Autodesk Inventor part; units mm, degrees
ref_plane "起始平面" through (0, 0, 0) normal (0, 1, 0) x (-1, 0, 0)
ref_plane "终止平面" through (0, 100, 0) normal (0, 1, 0) x (-1, 0, 0)
ref_plane "YZ Plane" through (0, 0, 0) normal (1, 0, 0) x (0, 1, 0)
ref_plane "起始平面" through (0, 0, 0) normal (0, 1, 0) x (-1, 0, 0)
ref_plane "终止平面" through (0, 100, 0) normal (0, 1, 0) x (-1, 0, 0)
sketch "草图" plane through (0, 0, 0) normal (0, 1, 0) x (-1, 0, 0)
  line L0 (-9.1, 10.0192) -> (-9.101, 10.0203)
  line L1 (-10, 10) -> (-9.5607, 9.5607) construction
  arc A0 (-8.5, 10) -> (-10, 8.5) centre (-8.5, 8.5) ccw
  circle A1 centre (0, 0) radius 2.5
  line L2 (-2.9808, 3.9) -> (0, 3.9)
  line L3 (-3.9, 0) -> (-3.9, 2.9808)
  line L4 (-2.5, 0) -> (-3.1, 0)
  line L5 (2.9808, 3.9) -> (0, 3.9)
  circle A2 centre (0, 0) radius 2.5
  circle A3 centre (0, 0) radius 2.5
  circle A4 centre (0, 0) radius 2.5
  line L6 (0, 16.3557) -> (0, -12.0006)
  line L7 (-4.3, 9.1) -> (-4.3, 10)
  line L8 (2.9808, -3.9) -> (0, -3.9)
  line L9 (-3.9, 0) -> (-3.9, -2.9808)
  line L10 (3.9, 0) -> (3.9, -2.9808)
  line L11 (-2.9808, -3.9) -> (-5.5, -6.4192)
  line L12 (-2.9808, -3.9) -> (0, -3.9)
  line L13 (3.8, -8.2) -> (3.8, -9.1)
  line L14 (5.5, -6.4192) -> (2.9808, -3.9)
  line L15 (3.8, -9.1) -> (4.3, -9.1)
  line L16 (5.5, -8.2) -> (3.8, -8.2)
  line L17 (5.5, -8.2) -> (5.5, -6.4192)
  line L18 (3.9, -2.9808) -> (6.4192, -5.5)
  line L19 (8.2, -3.8) -> (8.2, -5.5)
  line L20 (8.2, -5.5) -> (6.4192, -5.5)
  line L21 (8.2, -3.8) -> (9.1, -3.8)
  line L22 (9.1, -3.8) -> (9.1, -4.3)
  line L23 (9.1, -4.3) -> (10, -4.3)
  line L24 (10, -4.3) -> (10, -8.5)
  arc A5 (8.5, -10) -> (10, -8.5) centre (8.5, -8.5) ccw
  line L25 (8.5, -10) -> (4.3, -10)
  line L26 (4.3, -9.1) -> (4.3, -10)
  line L27 (5.5, 6.4192) -> (2.9808, 3.9)
  line L28 (3.9, 2.9808) -> (6.4192, 5.5)
  line L29 (10, 4.3) -> (10, 8.5)
  line L30 (3.9, 0) -> (3.9, 2.9808)
  line L31 (5.5, 8.2) -> (5.5, 6.4192)
  line L32 (5.5, 8.2) -> (3.8, 8.2)
  line L33 (4.3, 9.1) -> (4.3, 10)
  arc A6 (10, 8.5) -> (8.5, 10) centre (8.5, 8.5) ccw
  line L34 (8.5, 10) -> (4.3, 10)
  line L35 (8.2, 3.8) -> (9.1, 3.8)
  line L36 (9.1, 4.3) -> (10, 4.3)
  line L37 (9.1, 3.8) -> (9.1, 4.3)
  line L38 (8.2, 3.8) -> (8.2, 5.5)
  line L39 (8.2, 5.5) -> (6.4192, 5.5)
  line L40 (3.8, 8.2) -> (3.8, 9.1)
  line L41 (3.8, 9.1) -> (4.3, 9.1)
  line L42 (-10, 4.3) -> (-10, 8.5)
  line L43 (-8.5, 10) -> (-4.3, 10)
  line L44 (-9.1, 4.3) -> (-10, 4.3)
  line L45 (-9.1, 3.8) -> (-9.1, 4.3)
  line L46 (-8.2, 3.8) -> (-9.1, 3.8)
  line L47 (-8.2, 5.5) -> (-6.4192, 5.5)
  line L48 (-8.2, 3.8) -> (-8.2, 5.5)
  line L49 (-5.5, 8.2) -> (-5.5, 6.4192)
  line L50 (-3.8, 9.1) -> (-4.3, 9.1)
  line L51 (-3.8, 8.2) -> (-3.8, 9.1)
  line L52 (-5.5, 8.2) -> (-3.8, 8.2)
  line L53 (-3.9, 2.9808) -> (-6.4192, 5.5)
  line L54 (-2.9808, 3.9) -> (-5.5, 6.4192)
  line L55 (-5.5, -8.2) -> (-3.8, -8.2)
  line L56 (-5.5, -8.2) -> (-5.5, -6.4192)
  line L57 (-3.9, -2.9808) -> (-6.4192, -5.5)
  line L58 (-3.8, -8.2) -> (-3.8, -9.1)
  line L59 (-3.8, -9.1) -> (-4.3, -9.1)
  line L60 (-4.3, -9.1) -> (-4.3, -10)
  line L61 (-8.2, -5.5) -> (-6.4192, -5.5)
  line L62 (-8.2, -3.8) -> (-9.1, -3.8)
  line L63 (-9.1, -3.8) -> (-9.1, -4.3)
  line L64 (-8.5, -10) -> (-4.3, -10)
  line L65 (-9.1, -4.3) -> (-10, -4.3)
  line L66 (-10, -4.3) -> (-10, -8.5)
  arc A7 (-10, -8.5) -> (-8.5, -10) centre (-8.5, -8.5) ccw
  line L67 (-8.2, -3.8) -> (-8.2, -5.5)
  dimension "圆角" = 1.5
  dimension "宽度" = 20
extrude "实体" add sketch "草图" along normal up to surface (100 mm away) from surface at 0 contours L43 L7 L50 L51 L52 L49 L54 L2 L6 A1 L12 L11 L56 L55 L58 L59 L60 L64 A7 L66 L65 L63 L62 L67 L61 L57 L9 L3 L53 L47 L48 L46 L45 L44 L42 A0 | L5 L27 L31 L32 L40 L41 L33 L34 A6 L29 L36 L37 L35 L38 L39 L28 L30 L10 L18 L20 L19 L21 L22 L23 L24 A5 L25 L26 L15 L13 L16 L17 L14 L8 L6 A1
sketch "草图2" plane through (0, 0, 0) normal (0, 1, 0) x (-1, 0, 0)
  line L0 (0, 0) -> (10, 0)
ref_plane "工作平面3" through (0, 0, 0) normal (0, 0, -1) x (-1, 0, 0)
sketch "草图3" plane through (0, 0, 0) normal (0, 0, -1) x (-1, 0, 0)
  line L0 (-2, 0) -> (12, 0)
  line L1 (-2, 100) -> (12, 100)
  dimension "d11" = 100
equation "\"G_OFFSET_START\" = 0"
equation "\"G_OFFSET_END\" = 0"
equation "\"G_L\" = d11"
properties part number "欧标 2020铝合金钢材-01"
Can you work these out from the model? Positions are in its coordinate system, mm. A direction names the side the tool comes from. Give positions to 0.01 mm unless a question says otherwise; leave off trailing zeros. Write each loop counter-clockwise with the first axis right and the second up, starting at its lowest first coordinate (ties: lowest second). Pieces come first, ordered by that corner, then holes. Notation, with made-up numbers: (37, 58.25) -> (90, 58.25) arc R25 ccw to (90, 76.25) -> close; hole circle Ø3 at (56.5, 84). An arc over 180 degrees is marked (long way). Answer as a JSON object with one key per item and string values. Group by question number.
Item 1: For faces 1 (the face through (5.5, 49, -7)), 2 (the face through (10, 49, -6)), 3 (the face through (0, 49, -3.9)), 4 (the face through (-3.9, 49, 0)), which set-ups out of +Z, -Z, +X, -X, +Y, -Y let a thin tool reach every point of the face, with its end or its side?
Item 2: Suppose I cut it at B-B (x = 0). Please give me the cut outline in (y, z).
Item 3: Please list where these lines run through material, in increasing order: line 1 (X direction, y = 39.5, z = 0); line 2 (Z direction, x = 8.5, y = 89); line 3 (Z direction, x = 5.25, y = 60). Write a range as [from, to].
Item 4: I'm going to push flat-ended pins straight in: P1, Ø1.5, axis at y = 52.5, z = 1.5, coming from the -X side; P2, Ø2, axis at x = -3, z = 3.5, coming from the -Y side; P3, Ø5, axis at x = -1, y = 34.5, coming from the -Z side; P4, Ø0.5, axis at y = 27, z = -9.5, coming from the +X side. Where does each tip first touch, or does it pass through?
Item 5: We'd pull the mould along Z, two halves only. Please class faces 5 (the face through (-4.26, 49.3, 5.18)), 6 (the face through (-10, 49, -6)), 7 (the face through (0, 49, 3.9)): +Z half, -Z half, draft (parallel to the pull), parting line (faces both ways), or undercut.
Item 6: Suppose I cut it at A-A (z = 1.5). Please give me the cut outline in (x, y), plus the area to 3 significant figures.
Findings:
{
 "1": {"face 1": "+Y, -Y", "face 2": "+Z, -Z, +X, +Y, -Y", "face 3": "-Z, +Y, -Y", "face 4": "-X, +Y, -Y"},
 "2": {"outline": "(0, -3.9) -> (100, -3.9) -> (100, -2.5) -> (0, -2.5) -> close; (0, 2.5) -> (100, 2.5) -> (100, 3.9) -> (0, 3.9) -> close"},
 "3": {"line 1": "x = [-3.9, -2.5], [2.5, 3.9]", "line 2": "z = [-10, -3.8], [3.8, 10]", "line 3": "z = [-10, -8.2], [-6.17, -4.33], [4.33, 6.17], [8.2, 10]"},
 "4": {"P1": "stops at x = -3.9", "P2": "stops at y = 0", "P3": "stops at z = -4.42", "P4": "stops at x = 9.8"},
 "5": {"face 5": "undercut", "face 6": "draft", "face 7": "+Z half"},
 "6": {"outline": "(-3.9, 0) -> (-2, 0) -> (-2, 100) -> (-3.9, 100) -> close; (2, 0) -> (3.9, 0) -> (3.9, 100) -> (2, 100) -> close", "area": "380 mm²"}
}
